from build123d import *

# Parameters (mm, degrees)
VERTICAL_CARRIER_2MM_SKETCH_R  = 1.51
VERTICAL_CARRIER_2MM_DEPTH     = 2
INTEGRAL_FOOT_3MM_START        = 2
INTEGRAL_FOOT_3MM_SKETCH_W     = 36
INTEGRAL_FOOT_3MM_SKETCH_H     = 3
INTEGRAL_FOOT_3MM_DEPTH        = 11
FOOT_2X_D3P4_ISO273_START      = -28
FOOT_2X_D3P4_ISO273_SKETCH_R   = 1.7
FOOT_2X_D3P4_ISO273_DEPTH      = 3
BUCK_UNDERSIDE_RAILS_START     = 2
BUCK_UNDERSIDE_RAILS_SKETCH_W  = 31
BUCK_UNDERSIDE_RAILS_SKETCH_H  = 2
BUCK_UNDERSIDE_RAILS_DEPTH     = 1.65
BUCK_EDGE_GUIDES_START         = 2
BUCK_EDGE_GUIDES_SKETCH_W      = 31
BUCK_EDGE_GUIDES_SKETCH_H      = 1.2
BUCK_EDGE_GUIDES_DEPTH         = 3.55
BUCK_SLIDE_IN_LIPS_START       = 5.55
BUCK_SLIDE_IN_LIPS_SKETCH_W    = 31
BUCK_SLIDE_IN_LIPS_SKETCH_H    = 2.1
BUCK_SLIDE_IN_LIPS_DEPTH       = 1.05
RS485_UNDERSIDE_RAILS_START    = 2
RS485_UNDERSIDE_RAILS_SKETCH_W = 31
RS485_UNDERSIDE_RAILS_SKETCH_H = 2
RS485_UNDERSIDE_RAILS_DEPTH    = 1.65
RS485_EDGE_GUIDES_START        = 2
RS485_EDGE_GUIDES_SKETCH_W     = 31
RS485_EDGE_GUIDES_SKETCH_H     = 1.2
RS485_EDGE_GUIDES_DEPTH        = 3.55
RS485_SLIDE_IN_LIPS_START      = 5.55
RS485_SLIDE_IN_LIPS_SKETCH_W   = 31
RS485_SLIDE_IN_LIPS_SKETCH_H   = 2.1
RS485_SLIDE_IN_LIPS_DEPTH      = 1.05
PCB_INSERTION_STOPS_START      = 2
PCB_INSERTION_STOPS_DEPTH      = 3.3


with BuildPart() as part:
    # Vertical_carrier_2mm_Sketch → Vertical_carrier_2mm (new body)
    with BuildSketch(Plane.XY):
        with BuildLine():
            Line((-26, -28), (26, -28))
            ThreePointArc((26, -28), (27.767766953, -27.267766953), (28.5, -25.5))
            Line((28.5, -25.5), (28.5, 25.5))
            ThreePointArc((28.5, 25.5), (27.767766953, 27.267766953), (26, 28))
            Line((26, 28), (-26, 28))
            ThreePointArc((-26, 28), (-27.767766953, 27.267766953), (-28.5, 25.5))
            Line((-28.5, 25.5), (-28.5, -25.5))
            ThreePointArc((-28.5, -25.5), (-27.767766953, -27.267766953), (-26, -28))
        make_face()
        with Locations((-25.5, -23.5)):
            Circle(VERTICAL_CARRIER_2MM_SKETCH_R, mode=Mode.SUBTRACT)
        with Locations((18.6, -25.1)):
            Circle(VERTICAL_CARRIER_2MM_SKETCH_R, mode=Mode.SUBTRACT)
        with Locations((-25.5, 23.5)):
            Circle(VERTICAL_CARRIER_2MM_SKETCH_R, mode=Mode.SUBTRACT)
        with Locations((18.6, 25.1)):
            Circle(VERTICAL_CARRIER_2MM_SKETCH_R, mode=Mode.SUBTRACT)
    extrude(amount=VERTICAL_CARRIER_2MM_DEPTH)

    # Integral_foot_3mm_Sketch → Integral_foot_3mm (add)
    with BuildSketch(Plane.XY.offset(INTEGRAL_FOOT_3MM_START)):
        with Locations((-3, -26.5)):
            Rectangle(INTEGRAL_FOOT_3MM_SKETCH_W, INTEGRAL_FOOT_3MM_SKETCH_H)
    extrude(amount=INTEGRAL_FOOT_3MM_DEPTH)

    # Foot_2x_D3p4_ISO273_Sketch → Foot_2x_D3p4_ISO273 (cut)
    with BuildSketch(Plane(origin=(0, 0, 0), x_dir=(1, 0, 0), z_dir=(0, 1, 0)).offset(FOOT_2X_D3P4_ISO273_START)):
        with Locations(Location((-13, -10.9, 0), (0, 0, 270))):
            Circle(FOOT_2X_D3P4_ISO273_SKETCH_R)
        with Locations(Location((12, -10.9, 0), (0, 0, 270))):
            Circle(FOOT_2X_D3P4_ISO273_SKETCH_R)
    extrude(amount=FOOT_2X_D3P4_ISO273_DEPTH, mode=Mode.SUBTRACT)

    # Buck_underside_rails_Sketch → Buck_underside_rails (add)
    with BuildSketch(Plane.XY.offset(BUCK_UNDERSIDE_RAILS_START)):
        with Locations((0, 2)):
            Rectangle(BUCK_UNDERSIDE_RAILS_SKETCH_W, BUCK_UNDERSIDE_RAILS_SKETCH_H)
        with Locations((0, 22)):
            Rectangle(BUCK_UNDERSIDE_RAILS_SKETCH_W, BUCK_UNDERSIDE_RAILS_SKETCH_H)
    extrude(amount=BUCK_UNDERSIDE_RAILS_DEPTH)

    # Buck_edge_guides_Sketch → Buck_edge_guides (add)
    with BuildSketch(Plane.XY.offset(BUCK_EDGE_GUIDES_START)):
        with Locations((0, 0.7)):
            Rectangle(BUCK_EDGE_GUIDES_SKETCH_W, BUCK_EDGE_GUIDES_SKETCH_H)
        with Locations((0, 23.3)):
            Rectangle(BUCK_EDGE_GUIDES_SKETCH_W, BUCK_EDGE_GUIDES_SKETCH_H)
    extrude(amount=BUCK_EDGE_GUIDES_DEPTH)

    # Buck_slide_in_lips_Sketch → Buck_slide_in_lips (add)
    with BuildSketch(Plane.XY.offset(BUCK_SLIDE_IN_LIPS_START)):
        with Locations((0, 1.5)):
            Rectangle(BUCK_SLIDE_IN_LIPS_SKETCH_W, BUCK_SLIDE_IN_LIPS_SKETCH_H)
        with Locations((0, 22.5)):
            Rectangle(BUCK_SLIDE_IN_LIPS_SKETCH_W, BUCK_SLIDE_IN_LIPS_SKETCH_H)
    extrude(amount=BUCK_SLIDE_IN_LIPS_DEPTH)

    # RS485_underside_rails_Sketch → RS485_underside_rails (add)
    with BuildSketch(Plane.XY.offset(RS485_UNDERSIDE_RAILS_START)):
        with Locations((0, -21.5)):
            Rectangle(RS485_UNDERSIDE_RAILS_SKETCH_W, RS485_UNDERSIDE_RAILS_SKETCH_H)
        with Locations((0, -1.5)):
            Rectangle(RS485_UNDERSIDE_RAILS_SKETCH_W, RS485_UNDERSIDE_RAILS_SKETCH_H)
    extrude(amount=RS485_UNDERSIDE_RAILS_DEPTH)

    # RS485_edge_guides_Sketch → RS485_edge_guides (add)
    with BuildSketch(Plane.XY.offset(RS485_EDGE_GUIDES_START)):
        with Locations((0, -22.8)):
            Rectangle(RS485_EDGE_GUIDES_SKETCH_W, RS485_EDGE_GUIDES_SKETCH_H)
        with Locations((0, -0.2)):
            Rectangle(RS485_EDGE_GUIDES_SKETCH_W, RS485_EDGE_GUIDES_SKETCH_H)
    extrude(amount=RS485_EDGE_GUIDES_DEPTH)

    # RS485_slide_in_lips_Sketch → RS485_slide_in_lips (add)
    with BuildSketch(Plane.XY.offset(RS485_SLIDE_IN_LIPS_START)):
        with Locations((0, -22)):
            Rectangle(RS485_SLIDE_IN_LIPS_SKETCH_W, RS485_SLIDE_IN_LIPS_SKETCH_H)
        with Locations((0, -1)):
            Rectangle(RS485_SLIDE_IN_LIPS_SKETCH_W, RS485_SLIDE_IN_LIPS_SKETCH_H)
    extrude(amount=RS485_SLIDE_IN_LIPS_DEPTH)

    # PCB_insertion_stops_Sketch → PCB_insertion_stops (add)
    with BuildSketch(Plane.XY.offset(PCB_INSERTION_STOPS_START)):
        with BuildLine():
            Line((22.2, 4.5), (22.7, 4.5))
            ThreePointArc((22.7, 4.5), (22.947487373, 4.602512627), (23.05, 4.85))
            Line((23.05, 4.85), (23.05, 7.95))
            ThreePointArc((23.05, 7.95), (22.947487373, 8.197487373), (22.7, 8.3))
            Line((22.7, 8.3), (22.2, 8.3))
            ThreePointArc((22.2, 8.3), (21.952512627, 8.197487373), (21.85, 7.95))
            Line((21.85, 7.95), (21.85, 4.85))
            ThreePointArc((21.85, 4.85), (21.952512627, 4.602512627), (22.2, 4.5))
        make_face()
        with BuildLine():
            Line((24.2, -20.6), (24.7, -20.6))
            ThreePointArc((24.7, -20.6), (24.947487373, -20.497487373), (25.05, -20.25))
            Line((25.05, -20.25), (25.05, -17.65))
            ThreePointArc((25.05, -17.65), (24.947487373, -17.402512627), (24.7, -17.3))
            Line((24.7, -17.3), (24.2, -17.3))
            ThreePointArc((24.2, -17.3), (23.952512627, -17.402512627), (23.85, -17.65))
            Line((23.85, -17.65), (23.85, -20.25))
            ThreePointArc((23.85, -20.25), (23.952512627, -20.497487373), (24.2, -20.6))
        make_face()
    extrude(amount=PCB_INSERTION_STOPS_DEPTH)


solid = part.part
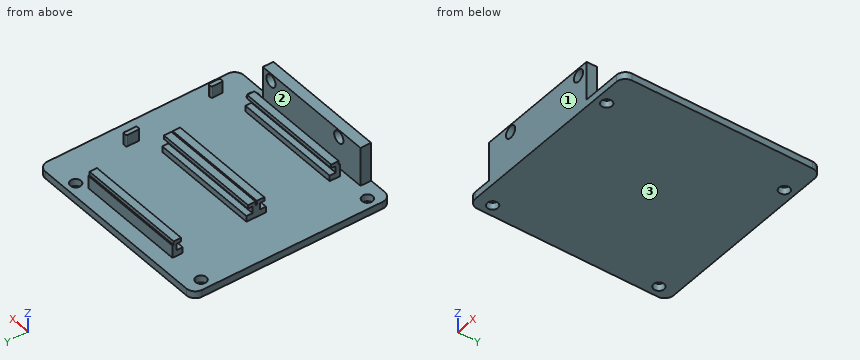
The listing builds one solid part. Answer for the finished solid, in the listing's coordinates (mm). Face numbers are marked on the shaded views. Coordinates: 2 decimals unless noted, no trailing zeros. Write each loop counter-clockwise with the first axis right and the second up, starting at its lowest first coordinate (ties: lowest second). Pieces come first, ordered by that corner, then holes. Notation, with made-up numbers: (29, 39) - (65, 39) arc R15 ccw to (65, 68) - close; hole circle Ø6 at (-6, 75). An arc over 180 degrees is marked (long way). Return JSON: item names as keys, results as strings.
1. For a pull along Y with two mould halves and no side action, classify the marked faces 1, 2 and 3 as +Y half, -Y half, draft (parallel to the pull), parting line (faces both ways), or undercut.
Final values:
{"face 1": "-Y half", "face 2": "undercut", "face 3": "draft"}
2. The part is cut by section B-B on x = -23. Determine the outline of the cut face in (y, z).
Final values:
{"outline": "(-28, 0) - (28, 0) - (28, 2) - (-28, 2) - close"}
3. The part is cut by section C-C on y = -4. Determine the outline of the cut face in (x, z), then the cut area to 3 significant figures.
Final values:
{"outline": "(-28.5, 0) - (28.5, 0) - (28.5, 2) - (-28.5, 2) - close", "area": "114 mm^2"}
4. The part is cut by section A-A on z = 10.9. Determine the outline of the cut face in (x, y).
Final values:
{"outline": "(-21, -28) - (-14.7, -28) - (-14.7, -25) - (-21, -25) - close; (-11.3, -28) - (10.3, -28) - (10.3, -25) - (-11.3, -25) - close; (13.7, -28) - (15, -28) - (15, -25) - (13.7, -25) - close"}
5. Each of these flat-tipped pins is pushed along its axis until it touches: pin 1 Ø0.5 at (x, y) = (0.5, -21) entering from +Z; pin 2 Ø4 at (x, z) = (-5, 3.5) entering from +Y; pin 3 Ø0.6 at (x, z) = (24.5, 4) entering from +Y; pin 4 Ø2.5 at (y, z) = (22.5, 3.5) entering from +X. Where does it stop, or does it pass through?
Final values:
{"pin 1": "z = 6.6", "pin 2": "y = 28", "pin 3": "y = -17.3", "pin 4": "x = 15.5"}
6. Consider line 1 along Y through (x, z) = (14, 4.5); line 2 along Y through (x, z) = (18.6, 0.55); line 3 along Y through (x, z) = (-25.5, 1.2). Determine where each line is inside the solid, lowest interval first.
Final values:
{"line 1": "-28 to -25, -23.4 to -22.2, -0.8 to 1.3, 22.7 to 23.9", "line 2": "-28 to -26.61, -23.59 to 23.59, 26.61 to 28", "line 3": "-28 to -25.01, -21.99 to 21.99, 25.01 to 28"}
